```python
from build123d import *

# Parameters (mm, degrees)
SKETCH1_W           = 10.67
SKETCH1_H           = 4.95
BOSS_EXTRUDE1_DEPTH = 8.3
SKETCH3_W           = 1.382324252
SKETCH3_H           = 1.382324252
CUT_EXTRUDE1_DEPTH  = 3
BOSS_EXTRUDE2_START = 3.31
BOSS_EXTRUDE2_DEPTH = 1
LPATTERN1_COUNT     = 4
LPATTERN1_PITCH     = 2.54
CHAMFER1_SIZE       = 0.25


with BuildPart() as part:
    # Sketch1 → Boss-Extrude1 (new body)
    with BuildSketch(Plane.XY):
        Rectangle(SKETCH1_W, SKETCH1_H)
    extrude(amount=BOSS_EXTRUDE1_DEPTH)

    # Sketch3 → Cut-Extrude1 (cut)
    with BuildSketch(Plane(origin=(0, 0, 0), x_dir=(-1, 0, 0), z_dir=(0, 0, -1))):
        with Locations((-1.27, 1.27)):
            Rectangle(SKETCH3_W, SKETCH3_H)
        with Locations((-3.81, 1.27)):
            Rectangle(SKETCH3_W, SKETCH3_H)
        with Locations((1.27, 1.27)):
            Rectangle(SKETCH3_W, SKETCH3_H)
        with Locations((3.81, 1.27)):
            Rectangle(SKETCH3_W, SKETCH3_H)
        with Locations((-1.27, -1.27)):
            Rectangle(SKETCH3_W, SKETCH3_H)
        with Locations((1.27, -1.27)):
            Rectangle(SKETCH3_W, SKETCH3_H)
        with Locations((3.81, -1.27)):
            Rectangle(SKETCH3_W, SKETCH3_H)
        with Locations((-3.81, -1.27)):
            Rectangle(SKETCH3_W, SKETCH3_H)
    extrude(amount=-CUT_EXTRUDE1_DEPTH, mode=Mode.SUBTRACT)

    # Sketch4 → Boss-Extrude2 (add)
    with BuildSketch(Plane(origin=(0, 0, 0), x_dir=(0, 0, -1), z_dir=(1, 0, 0)).offset(BOSS_EXTRUDE2_START)):
        with BuildLine():
            Line((-8.3, 0.77), (-9.32, 0.77))
            ThreePointArc((-9.32, 0.77), (-10.027106781, 1.062893219), (-10.32, 1.77))
            Line((-10.32, 1.77), (-10.32, 5.015))
            Line((-10.32, 5.015), (-9.32, 5.015))
            Line((-9.32, 5.015), (-9.32, 2.27))
            ThreePointArc((-9.32, 2.27), (-9.173553391, 1.916446609), (-8.82, 1.77))
            Line((-8.82, 1.77), (-8.3, 1.77))
            Line((-8.3, 1.77), (-8.3, 0.77))
        make_face()
        with BuildLine():
            Line((-8.3, -1.77), (-11.86, -1.77))
            ThreePointArc((-11.86, -1.77), (-12.567106781, -1.477106781), (-12.86, -0.77))
            Line((-12.86, -0.77), (-12.86, 5.015))
            Line((-12.86, 5.015), (-11.86, 5.015))
            Line((-11.86, 5.015), (-11.86, -0.27))
            ThreePointArc((-11.86, -0.27), (-11.713553391, -0.623553391), (-11.36, -0.77))
            Line((-11.36, -0.77), (-8.3, -0.77))
            Line((-8.3, -0.77), (-8.3, -1.77))
        make_face()
    boss_extrude2 = extrude(amount=BOSS_EXTRUDE2_DEPTH)

    # LPattern1: Boss-Extrude2 ×4
    with Locations(*[(-i * LPATTERN1_PITCH, 0, 0) for i in range(1, LPATTERN1_COUNT)]):
        add(boss_extrude2)

    # Chamfer1
    chamfer1_edges = [part.edges().sort_by_distance(p)[0] for p in [
        (3.31, 5.015, 9.82),
        (3.81, 5.015, 9.32),
        (3.81, 5.015, 10.32),
        (4.31, 5.015, 9.82),
        (3.31, 5.015, 12.36),
        (3.81, 5.015, 11.86),
        (3.81, 5.015, 12.86),
        (4.31, 5.015, 12.36),
        (0.77, 5.015, 9.82),
        (1.27, 5.015, 9.32),
        (1.27, 5.015, 10.32),
        (1.77, 5.015, 9.82),
        (0.77, 5.015, 12.36),
        (1.27, 5.015, 11.86),
        (1.27, 5.015, 12.86),
        (1.77, 5.015, 12.36),
        (-1.77, 5.015, 9.82),
        (-1.27, 5.015, 9.32),
        (-1.27, 5.015, 10.32),
        (-0.77, 5.015, 9.82),
        (-1.77, 5.015, 12.36),
        (-1.27, 5.015, 11.86),
        (-1.27, 5.015, 12.86),
        (-0.77, 5.015, 12.36),
        (-4.31, 5.015, 9.82),
        (-3.81, 5.015, 9.32),
        (-3.81, 5.015, 10.32),
        (-3.31, 5.015, 9.82),
        (-4.31, 5.015, 12.36),
        (-3.81, 5.015, 11.86),
        (-3.81, 5.015, 12.86),
        (-3.31, 5.015, 12.36),
    ]]
    chamfer(chamfer1_edges, length=CHAMFER1_SIZE)


solid = part.part
```
The listing builds one solid part. Answer for the finished solid, in the listing's coordinates (mm). A direction names the side the tool comes from. Round coordinates to 2 decimals unless told otherwise and drop trailing zeros. Loops run counter-clockwise (first coordinate to the right, second up) from the corner with the lowest first, then second, coordinate; pieces in that order, holes last.
Q1. Section C-C, the plane y = 4 is taken. Count the separate pieces of the cut face and the enclosed holes in it, then the cut area to 3 significant figures.
Q2. Find the intervals of material crossed by line 1 (X direction, y = 2.5, z = 10); line 2 (X direction, y = 0.75, z = 0.75) (3 decimals); line 3 (Y direction, x = -3.5, z = 2.5) (3 decimals), in increasing order.
Q3. Section A-A, the plane y = 0 is taken. Determine the outline of the cut face in (x, z) (3 decimals), then the cut area to 3 significant figures.
Q4. For a pull along Z with two mould halves and no side action, classify faces 1 (the face through (3.119, -1, 1)), 2 (the face through (4, 3, 10.32)), 3 (the face through (4, 2, 12.86)) as released by +Z, released by -Z, zero draft, split by the parting line, or undercut.
Q5. Given pin 1 Ø1 at (x, z) = (0.5, 7) entering from +Y (3 decimals); pin 2 Ø2 at (y, z) = (0, 11) entering from +X; pin 3 Ø0.5 at (x, y) = (-1.5, 3.5) entering from -Z, each flat-ended and moving along its own axis, determine where each tip first touches the part or whether it passes through.
Q6. Which of the six approach directions +Z, -Z, +X, -X, +Y, -Y give full straight-line access (tool end or side, diameter ignored) to faces 4 (the face through (-1, 1, 3)), 5 (the face through (-4.31, 0.8, 12.1)), 6 (the face through (0.77, 2, 10)), 7 (the face through (-1.277, 1.055, 10.019)), 8 (the face through (0, 0, 8.3))?
Q7. Section B-B, the plane z = 10.5 is taken. Determine the outline of the cut face in (x, y).
Completed:
1. separate pieces: 8
1. enclosed holes: 0
1. area: 8.00 mm2
2. line 1: x = -4.31 to -3.31, -1.77 to -0.77, 0.77 to 1.77, 3.31 to 4.31
2. line 2: x = -5.335 to -4.501, -3.119 to -1.961, -0.579 to 0.579, 1.961 to 3.119, 4.501 to 5.335
2. line 3: y = -2.475 to -1.961, -0.579 to 0.579, 1.961 to 2.475
3. outline: (-5.335, 0) - (5.335, 0) - (5.335, 8.3) - (-5.335, 8.3) - close; (-4.31, 11.86) - (-3.31, 11.86) - (-3.31, 12.86) - (-4.31, 12.86) - close; (-1.77, 11.86) - (-0.77, 11.86) - (-0.77, 12.86) - (-1.77, 12.86) - close; (0.77, 11.86) - (1.77, 11.86) - (1.77, 12.86) - (0.77, 12.86) - close; (3.31, 11.86) - (4.31, 11.86) - (4.31, 12.86) - (3.31, 12.86) - close
3. area: 92.6 mm2
4. face 1: zero draft
4. face 2: undercut
4. face 3: released by +Z
5. pin 1: stops at y = 2.475
5. pin 2: stops at x = 4.31
5. pin 3: stops at z = 9.32
6. face 4: -Z
6. face 5: +Z, -X, +Y, -Y
6. face 6: +Z, +Y, -Y
6. face 7: +X, -X
6. face 8: none
7. outline: (-4.31, -1.77) - (-3.31, -1.77) - (-3.31, -0.77) - (-4.31, -0.77) - close; (-1.77, -1.77) - (-0.77, -1.77) - (-0.77, -0.77) - (-1.77, -0.77) - close; (0.77, -1.77) - (1.77, -1.77) - (1.77, -0.77) - (0.77, -0.77) - close; (3.31, -1.77) - (4.31, -1.77) - (4.31, -0.77) - (3.31, -0.77) - close
